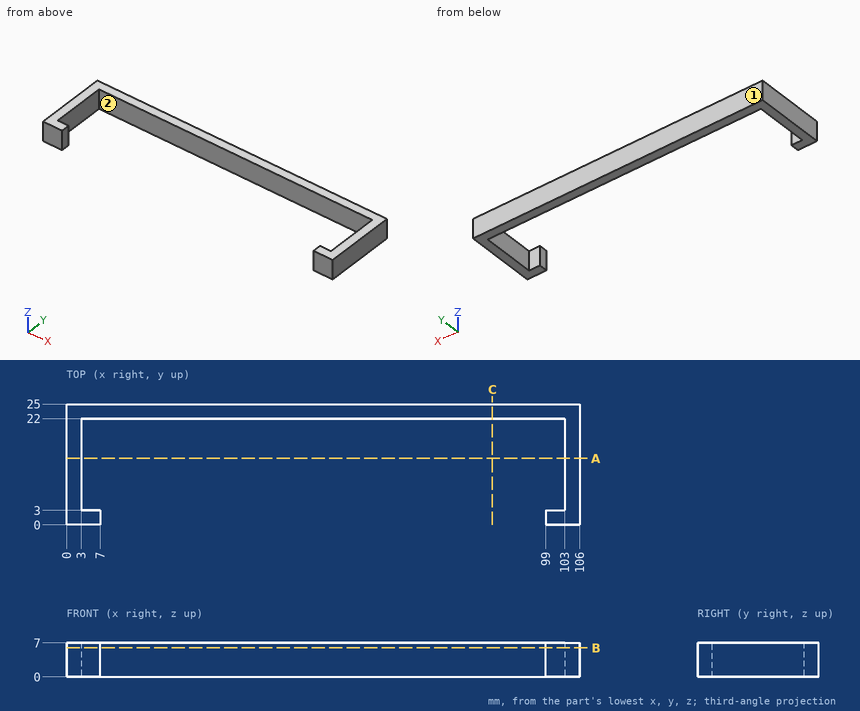
Source: three-view drawing plus pictorial views. Frame: mm from the lowest corner of the part. Coordinates: 2 decimals unless noted, no trailing zeros. Order: outer loops, then holes, each group sorted by start corner. A loop starts at its lowest first (then second) coordinate and runs counter-clockwise, first axis right, second up.
Item 1: Cut plane A-A (y = 13.75). Return loops of the section in (x, z).
Output values:
outline: (0, 0) - (3, 0) - (3, 7) - (0, 7) - close; (103, 0) - (106, 0) - (106, 7) - (103, 7) - close
Item 2: First-contact query: P1, Ø2.5, axis at y = 1.5, z = 5, coming from the -X side; P2, Ø2, axis at x = 62.5, z = 2, coming from the -Y side. Flat tips, straight axial feed; report the tip coordinate or a pass-through.
Output values:
P1: stops at x = 0
P2: stops at y = 22
Item 3: Cut plane C-C (x = 88). Return loops of the section in (y, z), plus the area to 3 significant figures.
Output values:
outline: (22, 0) - (25, 0) - (25, 7) - (22, 7) - close
area: 21.0 mm2
Item 4: Cut plane B-B (z = 6). Return loops of the section in (x, y), plus the area to 3 significant figures.
Output values:
outline: (0, 0) - (7, 0) - (7, 3) - (3, 3) - (3, 22) - (103, 22) - (103, 3) - (99, 3) - (99, 0) - (106, 0) - (106, 25) - (0, 25) - close
area: 474 mm2
Item 5: Pull-direction query (X, two-part tool) for the marked faces 1 and 2; classes: pulls with the +X half, pulls with the -X half, needs draft (parallel to the pull), parting line crosses it, or undercut.
Output values:
face 1: needs draft
face 2: undercut
Item 6: Material intervals for line 1 (X direction, y = 12, z = 0.75); line 2 (Y direction, x = 61.5, z = 5), sorted ascending.
Output values:
line 1: x = 0 to 3, 103 to 106
line 2: y = 22 to 25
